Can you work these out from the model? Positions are in its coordinate system, mm. A direction names the side the tool comes from. Give positions to 0.01 mm unless a question says otherwise; leave off trailing zeros. Loops run counter-clockwise (first coordinate to the right, second up) from the corner with the lowest first, then second, coordinate; pieces in that order, holes last. Notation, with made-up numbers: (-34.75, -18.75) - (13.25, -18.75) arc R22 cw to (13.25, -0.75) - close; hole circle Ø4 at (41, -6). An arc over 180 degrees is marked (long way). Answer in a Markdown table with one row per item.
from build123d import *

# Parameters (mm, degrees)
SKETCH_1_W          = 240
SKETCH_1_H          = 270
EXTRUDE_1_DEPTH     = 12
SKETCH_2_W          = 270
SKETCH_2_H          = 100
EXTRUDE_2_DEPTH     = 12
SKETCH_3_W          = 12
SKETCH_3_H          = 78
EXTRUDE_3_DEPTH     = 240
SKETCH_4_R          = 13
CUT_EXTRUDE_1_DEPTH = 361.898877804
SKETCH_5_R          = 13
CUT_EXTRUDE_2_DEPTH = 378.475827041


with BuildPart() as part:
    # 草图1 → 凸台-拉伸1 (new body)
    with BuildSketch(Plane(origin=(0, 0, 0), x_dir=(1, 0, 0), z_dir=(0, 1, 0))):
        with Locations((120, 135)):
            Rectangle(SKETCH_1_W, SKETCH_1_H)
    extrude(amount=EXTRUDE_1_DEPTH)

    # 草图2 → 凸台-拉伸2 (add)
    with BuildSketch(Plane.ZY):
        with Locations((-135, -28)):
            Rectangle(SKETCH_2_W, SKETCH_2_H)
    extrude(amount=EXTRUDE_2_DEPTH)

    # 草图3 → 凸台-拉伸3 (add)
    with BuildSketch(Plane(origin=(0, 0, 0), x_dir=(0, 0, -1), z_dir=(1, 0, 0))):
        with Locations((264, -39)):
            Rectangle(SKETCH_3_W, SKETCH_3_H)
    extrude(amount=EXTRUDE_3_DEPTH)

    # 草图4 → 切除-拉伸1 (cut, through all)
    with BuildSketch(Plane.XY.offset(-258)):
        with Locations((82, -38)):
            Circle(SKETCH_4_R)
        with Locations((202, -38)):
            Circle(SKETCH_4_R)
    extrude(amount=-CUT_EXTRUDE_1_DEPTH, mode=Mode.SUBTRACT)

    # 草图5 → 切除-拉伸2 (cut, through all)
    with BuildSketch(Plane.ZY.offset(12)):
        with Locations((-217, -38)):
            Circle(SKETCH_5_R)
        with Locations((-137, -38)):
            Circle(SKETCH_5_R)
        Polygon((-100, -78), (0, 0), (0, -78), align=None)
    extrude(amount=-CUT_EXTRUDE_2_DEPTH, mode=Mode.SUBTRACT)


solid = part.part
Q1. If I drill on line 1 (Y direction, x = 82, z = -265.25); line 2 (Y direction, x = -4.75, z = -217); line 3 (Y direction, x = 49, z = -54), over which ranges is the centre line in solid material (lowest first)? Write a range as [from, to].
Checked values:
| item | result |
|---|---|
| line 1 | y = [-78, -51], [-25, 12] |
| line 2 | y = [-78, -51], [-25, 22] |
| line 3 | y = [0, 12] |
Q2. Imagine slicing it at C-C, the plane y = -44. Write out the boundary of the cut face in (x, z).
Checked values:
| item | result |
|---|---|
| outline | (-12, -270) - (70.47, -270) - (70.47, -258) - (0, -258) - (0, -228.53) - (-12, -228.53) - close; (-12, -205.47) - (0, -205.47) - (0, -148.53) - (-12, -148.53) - close; (-12, -125.47) - (0, -125.47) - (0, -56.41) - (-12, -56.41) - close; (93.53, -270) - (190.47, -270) - (190.47, -258) - (93.53, -258) - close; (213.53, -270) - (240, -270) - (240, -258) - (213.53, -258) - close |
Q3. If we mould it in two halves opening along Y, with no side actions, what happens to faces 4 (the face through (-6, 22, -137)), 5 (the face through (-6.1, -34.1, -124.6)), 6 (the face through (69.013, -37.428, -263.916)), 7 (the face through (0, 17, -137))? For each: released by +Y, released by -Y, zero draft, split by the parting line, or undercut.
Checked values:
| item | result |
|---|---|
| face 4 | released by +Y |
| face 5 | undercut |
| face 6 | undercut |
| face 7 | zero draft |
Q4. On a 3-axis mill with a long thin cutter (end or side, diameter ignored), from which of +Z, -Z, +X, -X, +Y, -Y can I reach the whole of each face in a straight line? I mean faces 1 (the face through (118, -40, -258)), 2 (the face through (118, 12, -137)), 3 (the face through (76, -78, -260)). Say none if no direction works.
Checked values:
| item | result |
|---|---|
| face 1 | +Z, +X, -Y |
| face 2 | +Z, -Z, +X, +Y |
| face 3 | +Z, -Z, +X, -X, -Y |
Q5. Imagine slicing it at D-D, the plane z = -37. Write out the boundary of the cut face in (x, y).
Checked values:
| item | result |
|---|---|
| outline | (-12, -28.86) - (0, -28.86) - (0, 0) - (240, 0) - (240, 12) - (0, 12) - (0, 22) - (-12, 22) - close |
Q6. Imagine slicing it at B-B, the plane z = -217. Write out the boundary of the cut face in (x, y).
Checked values:
| item | result |
|---|---|
| outline | (-12, -78) - (0, -78) - (0, -51) - (-12, -51) - close; (-12, -25) - (0, -25) - (0, 0) - (240, 0) - (240, 12) - (0, 12) - (0, 22) - (-12, 22) - close |
Q7. Imagine slicing it at A-A, the plane x = 82. Write out the boundary of the cut face in (y, z), and give its area (3 significant figures).
Checked values:
| item | result |
|---|---|
| outline | (-78, -270) - (-51, -270) - (-51, -258) - (-78, -258) - close; (-25, -270) - (12, -270) - (12, 0) - (0, 0) - (0, -258) - (-25, -258) - close |
| area | 3,860 mm² |
Q8. For pin 1 (1.5 mm diameter, centred on x = 207.5, y = -53, fed in from +Z); pin 2 (3 mm diameter, centred on x = 93.5, z = -103.5, fed in from +Y); pin 3 (23.5 mm diameter, centred on y = -38, z = -137, fed in from -X); pin 4 (1 mm diameter, centred on y = -60.5, z = -94.5, fed in from +X), each with a flat end and sliding along its axis, tell me the tip position at first contact or that it passes through.
Checked values:
| item | result |
|---|---|
| pin 1 | stops at z = -258 |
| pin 2 | stops at y = 12 |
| pin 3 | passes through |
| pin 4 | stops at x = 0 |
